```python
from build123d import *

# Parameters (mm, degrees)
SKETCH1_W           = 19.05
SKETCH1_H           = 7.62
BOSS_EXTRUDE1_DEPTH = 1.905
SKETCH2_R           = 3.175
BOSS_EXTRUDE2_DEPTH = 5.715
SKETCH3_W           = 1.905
SKETCH3_H           = 7.62
BOSS_EXTRUDE3_DEPTH = 5.715


with BuildPart() as part:
    # Sketch1 → Boss-Extrude1 (new body)
    with BuildSketch(Plane(origin=(0, 0, 0), x_dir=(-1, 0, 0), z_dir=(0, 1, 0))):
        with Locations((9.525, 3.81)):
            Rectangle(SKETCH1_W, SKETCH1_H)
    extrude(amount=BOSS_EXTRUDE1_DEPTH)

    # Sketch2 → Boss-Extrude2 (add)
    with BuildSketch(Plane(origin=(0, 1.905, 0), x_dir=(-1, 0, 0), z_dir=(0, 1, 0))):
        with Locations(Location((9.525, 3.81, 0), (0, 0, 90))):
            Circle(SKETCH2_R)
    extrude(amount=BOSS_EXTRUDE2_DEPTH)

    # Sketch3 → Boss-Extrude3 (add)
    with BuildSketch(Plane(origin=(0, 1.905, 0), x_dir=(-1, 0, 0), z_dir=(0, 1, 0))):
        with Locations((0.9525, 3.81)):
            Rectangle(SKETCH3_W, SKETCH3_H)
        with Locations((18.0975, 3.81)):
            Rectangle(SKETCH3_W, SKETCH3_H)
    extrude(amount=BOSS_EXTRUDE3_DEPTH)


solid = part.part
```
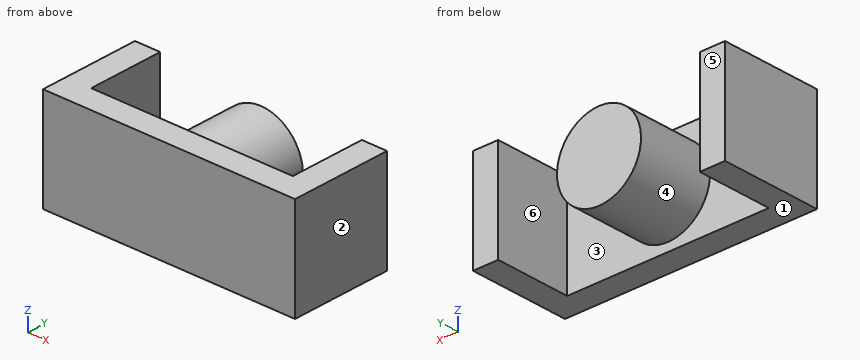
Input: part model. Units: mm. Frame: model coordinates. Face numbers are marked on the shaded views. A direction names the side the tool comes from. Round coordinates to 2 decimals unless told otherwise and drop trailing zeros. Write each loop counter-clockwise with the first axis right and the second up, starting at its lowest first coordinate (ties: lowest second). Pieces come first, ordered by that corner, then holes. Notation, with made-up numbers: M 26.25,51.5 L 41.25,51.5 A14 cw 41.25,73.5 Z; hole C 13.5,-9.75 d6. An arc over 180 degrees is marked long. Write each question's results on one line, items separated by ' | '.
Q1. Section query C-C (x = -8). Return loops of the section in (y, z) (3 decimals), and give its area (3 significant figures).
Results:
outline: M 0,0 L 1.905,0 L 1.905,1.025 L 7.62,1.025 L 7.62,6.595 L 1.905,6.595 L 1.905,7.62 L 0,7.62 Z | area: 46.3 mm^2
Q2. Section query D-D (z = 6.5). Return loops of the section in (x, y) (3 decimals).
Results:
outline: M -19.05,0 L 0,0 L 0,7.62 L -1.905,7.62 L -1.905,1.905 L -7.838,1.905 L -7.838,7.62 L -11.212,7.62 L -11.212,1.905 L -17.145,1.905 L -17.145,7.62 L -19.05,7.62 Z
Q3. Draft query along X for the marked faces 1, 2 and 3. Return one class per face: released by +X, released by -X, zero draft, split by the parting line, or undercut.
Results:
face 1: zero draft | face 2: released by +X | face 3: undercut
Q4. Line query: line 1 along X through (y, z) = (7, 1.25) (3 decimals); line 2 along X through (y, z) = (3, 1) (3 decimals); line 3 along Y through (x, z) = (-14, 4.75) (3 decimals). Output: solid intervals per line, ascending.
Results:
line 1: x = -19.05 to -17.145, -11.403 to -7.647, -1.905 to 0 | line 2: x = -19.05 to -17.145, -11.003 to -8.047, -1.905 to 0 | line 3: y = 0 to 1.905
Q5. Section query B-B (y = 4). Return loops of the section in (x, z) (3 decimals), and give its area (3 significant figures).
Results:
outline: M -19.05,0 L -17.145,0 L -17.145,7.62 L -19.05,7.62 Z; C -9.525,3.81 d6.35; M -1.905,0 L 0,0 L 0,7.62 L -1.905,7.62 Z | area: 60.7 mm^2
Q6. Access query for the marked faces 4, 5 and 6. Directions: +Z, -Z, +X, -X, +Y, -Y. A direction counts if a zero-diameter tool reaches every point of the face in a straight line with its end or side. Return the directions, or none.
Results:
face 4: +Y | face 5: +Z, -Z, +X, -X, +Y | face 6: +Z, -Z, +Y
Q7. Section query A-A (z = 3.81). Return loops of the section in (x, y) (3 decimals).
Results:
outline: M -19.05,0 L 0,0 L 0,7.62 L -1.905,7.62 L -1.905,1.905 L -6.35,1.905 L -6.35,7.62 L -12.7,7.62 L -12.7,1.905 L -17.145,1.905 L -17.145,7.62 L -19.05,7.62 Z
Q8. Pin query (flat end, axial travel): P1, Ø1, axis at x = -2, y = 4, coming from the -Z side. Return the tip coordinate at first contact, or that it passes through.
Results:
P1: stops at z = 0
